Geometry: final body of the model. Coordinates: model frame, mm. Coordinates: 2 decimals unless noted, no trailing zeros. Order: outer loops, then holes, each group sorted by start corner. A loop starts at its lowest first (then second) coordinate and runs counter-clockwise, first axis right, second up. Notation, with made-up numbers: (-29.75, 28) -> (20.25, 28) arc R17 cw to (20.25, 58) -> close; hole circle Ø8 at (67, 22.5). An arc over 180 degrees is marked (long way). Use one line per item in the form item = value.
```python
from build123d import *

# Parameters (mm, degrees)
F0_W           = 12.7
F0_H           = 12.7
F1_DEPTH       = 304.8
F3_D           = 4.318
F3_CSINK_D     = 9.1186
F3_CSINK_ANGLE = 82


with BuildPart() as f1:
    # F0 (on Front) → F1 (new body)
    with BuildSketch(Plane.XZ):
        with Locations((6.35, 6.35)):
            Rectangle(F0_W, F0_H)
    extrude(amount=F1_DEPTH)

    # F3 (through all)
    with Locations(Plane.XY.offset(12.7)):
        with Locations((6.35, -9.525), (6.35, -122.555), (6.35, -235.585), (6.35, -279.4), (6.35, -295.275)):
            CounterSinkHole(F3_D / 2, F3_CSINK_D / 2, counter_sink_angle=F3_CSINK_ANGLE)


solid = f1.part
```
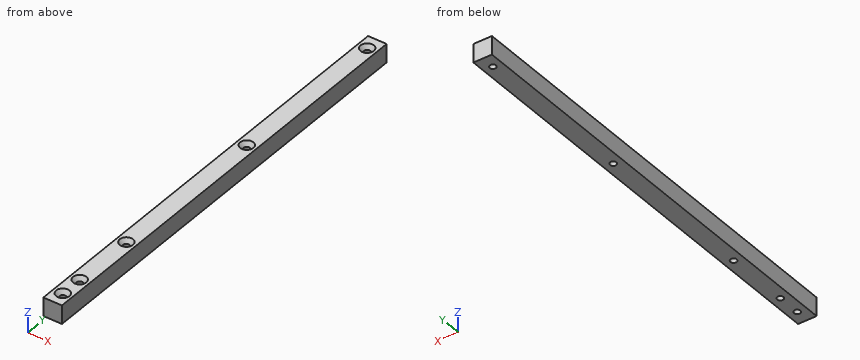
1) Section A-A, the plane x = 6.35. Give the number of separate pieces and of enclosed holes in the cut face, and give its area (3 significant figures).
Results found:
separate_pieces = 6
enclosed_holes = 0
area = 3,560 mm2
2) Material intervals for probe 1 along Y at (x, z) = (6.25, 8); probe 2 along X at (y, z) = (-279.4, 6); probe 3 along Y at (x, z) = (6, 10.75), sorted ascending. Write a range as from..to.
Results found:
probe_1 = -304.8..-297.43, -293.12..-281.56, -277.24..-237.74, -233.43..-124.71, -120.4..-11.68, -7.37..0
probe_2 = 0..4.19, 8.51..12.7
probe_3 = -304.8..-298.12, -292.43..-282.24, -276.56..-238.43, -232.74..-125.4, -119.71..-12.37, -6.68..0
3) Contact query for flat-ended pins moving along their axis: P1, Ø2.5, axis at x = 6.35, y = -295.275, coming from the +Z side; P2, Ø5, axis at y = -198, z = 3.5, coming from the -X side. Output: stop coordinate, or through.
Results found:
P1 = through
P2 = 0
4) Section B-B, the plane z = 6. Output: boundary loops of the cut face in (x, y) (3 decimals), and give its area (3 significant figures).
Results found:
outline = (0, -304.8) -> (12.7, -304.8) -> (12.7, 0) -> (0, 0) -> close; hole circle Ø4.318 at (6.35, -295.275); hole circle Ø4.318 at (6.35, -279.4); hole circle Ø4.318 at (6.35, -235.585); hole circle Ø4.318 at (6.35, -122.555); hole circle Ø4.318 at (6.35, -9.525)
area = 3,800 mm2
